Geometry: final body of the model. Coordinates: model frame, mm. Give positions to 0.01 mm unless a question says otherwise; leave off trailing zeros. Write each loop counter-clockwise with the first axis right and the second up, starting at its lowest first coordinate (ties: lowest second). Pieces come first, ordered by that corner, then holes. Notation, with made-up numbers: M 50,-13 L 104,-13 A32 ccw 104,23 Z; hole C 82,20 d7. An arc over 180 degrees is marked long. Use a Markdown table: item, result. Add a question column.
1) Section B-B on z = -6.5. Return the cut outline in (x, y) (3 decimals), then the cut area to 3 significant figures.
2) Section A-A on z = 1.75. Return the cut outline in (x, y) (3 decimals), then the cut area to 3 significant figures.
3) Line query: line 1 (Y direction, x = -11.5, z = 0.25); line 2 (Z direction, x = 7.25, y = -1); line 3 (Z direction, x = -9.5, y = 12.25). Output: solid intervals per line, ascending.
4) Pin query (flat end, axial travel): pin 1 (5 mm diameter, centred on y = 11, z = -1.5, fed in from -X); pin 2 (4 mm diameter, centred on x = -9, y = 8.5, fed in from -Z); pin 3 (1.4 mm diameter, centred on x = 10.5, z = 2, fed in from +Y); pin 4 (0.7 mm diameter, centred on y = -12.5, z = -1, fed in from -X). Return the tip coordinate at first contact, or that it passes through.
5) Section C-C on y = -3.5. Return the cut outline in (x, z).
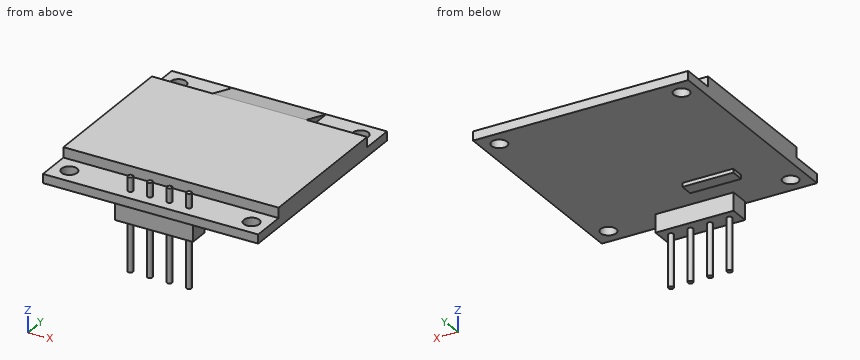
```python
from build123d import *

# Parameters (mm, degrees)
ESQUISSE1_W                = 27.56
ESQUISSE1_H                = 27.82
ESQUISSE1_R                = 1
BOSS_EXTRU_1_DEPTH         = 1.15
ESQUISSE3_W                = 27.56
ESQUISSE3_H                = 19.1
BOSS_EXTRU_2_DEPTH         = 1.3
BOSS_EXTRU_3_START         = -10.1
ESQUISSE4_R                = 0.325
BOSS_EXTRU_3_DEPTH         = 11.9
R_P_TITION_LIN_AIRE1_COUNT = 4
R_P_TITION_LIN_AIRE1_PITCH = 2.5
ESQUISSE5_W                = 6.517687079
ESQUISSE5_H                = 1.70105674
BOSS_EXTRU_4_DEPTH         = 0.5
ESQUISSE6_W                = 10
ESQUISSE6_H                = 2.5
BOSS_EXTRU_5_DEPTH         = 2.3
BOSS_EXTRU_6_DEPTH         = 6


with BuildPart() as part:
    # Esquisse1 → Boss.-Extru.1 (new body)
    with BuildSketch(Plane.XY):
        Rectangle(ESQUISSE1_W, ESQUISSE1_H)
        with Locations((-11.668662175, 11.778743894)):
            Circle(ESQUISSE1_R, mode=Mode.SUBTRACT)
        with Locations((11.668662175, 11.778743894)):
            Circle(ESQUISSE1_R, mode=Mode.SUBTRACT)
        with Locations((-11.668662175, -11.778743894)):
            Circle(ESQUISSE1_R, mode=Mode.SUBTRACT)
        with Locations((11.668662175, -11.778743894)):
            Circle(ESQUISSE1_R, mode=Mode.SUBTRACT)
    extrude(amount=BOSS_EXTRU_1_DEPTH)

    # Esquisse3 → Boss.-Extru.2 (add)
    with BuildSketch(Plane.XY.offset(1.15)):
        with Locations((0, 0.06)):
            Rectangle(ESQUISSE3_W, ESQUISSE3_H)
    extrude(amount=BOSS_EXTRU_2_DEPTH)

    # Esquisse4 → Boss.-Extru.3 (add)
    with BuildSketch(Plane.XY.offset(1.15).offset(BOSS_EXTRU_3_START)):
        with Locations((-3.53, -12.31)):
            Circle(ESQUISSE4_R)
    boss_extru_3 = extrude(amount=BOSS_EXTRU_3_DEPTH)

    # Répétition linéaire1: Boss.-Extru.3 ×4
    with Locations(*[(i * R_P_TITION_LIN_AIRE1_PITCH, 0, 0) for i in range(1, R_P_TITION_LIN_AIRE1_COUNT)]):
        add(boss_extru_3)

    # Esquisse5 → Boss.-Extru.4 (add)
    with BuildSketch(Plane(origin=(0, 0, 0), x_dir=(-1, 0, 0), z_dir=(0, 0, -1))):
        with Locations((4.307160535, -7.158796769)):
            Rectangle(ESQUISSE5_W, ESQUISSE5_H)
    extrude(amount=BOSS_EXTRU_4_DEPTH)

    # Esquisse6 → Boss.-Extru.5 (add)
    with BuildSketch(Plane(origin=(0, 0, 0), x_dir=(-1, 0, 0), z_dir=(0, 0, -1))):
        with Locations((-0.22, -12.31)):
            Rectangle(ESQUISSE6_W, ESQUISSE6_H)
    extrude(amount=BOSS_EXTRU_5_DEPTH)

    # Esquisse7 → Boss.-Extru.6 (add, symmetric)
    with BuildSketch(Plane(origin=(0, 0, 0), x_dir=(0, 0, -1), z_dir=(1, 0, 0))):
        Polygon((-1.15, 13.91), (-2.45, 9.61), (-1.15, 9.61), align=None)
    extrude(amount=BOSS_EXTRU_6_DEPTH, both=True)


solid = part.part
```
Found:
| question | item | result |
|---|---|---|
| 1 | outline | C -3.53,-12.31 d0.65; C -1.03,-12.31 d0.65; C 1.47,-12.31 d0.65; C 3.97,-12.31 d0.65 |
| 1 | area | 1.33 mm² |
| 2 | outline | M -13.78,-9.49 L 13.78,-9.49 L 13.78,9.61 L 6,9.61 L 6,11.925 L -6,11.925 L -6,9.61 L -13.78,9.61 Z; C -3.53,-12.31 d0.65; C -1.03,-12.31 d0.65; C 1.47,-12.31 d0.65; C 3.97,-12.31 d0.65 |
| 2 | area | 556 mm² |
| 3 | line 1 | -13.91 to -12.76, -10.79 to 10.79, 12.76 to 13.91 |
| 3 | line 2 | 0 to 2.45 |
| 3 | line 3 | 0 to 1.15 |
| 4 | pin 1 | x = -13.78 |
| 4 | pin 2 | z = 0 |
| 4 | pin 3 | y = 9.61 |
| 4 | pin 4 | x = -4.78 |
| 5 | outline | M -13.78,0 L 13.78,0 L 13.78,2.45 L -13.78,2.45 Z |
